Here's how the part is built. I have some questions about the finished solid (model axes, mm). A direction names the side the tool comes from. Round coordinates to 2 decimals unless told otherwise and drop trailing zeros. Loops run counter-clockwise (first coordinate to the right, second up) from the corner with the lowest first, then second, coordinate; pieces in that order, holes last. Notation, with made-up numbers: (54, 9.25) -> (69, 9.25) arc R17 cw to (69, 33.25) -> close; hole circle Ø6 at (28.5, 6). An arc over 180 degrees is marked (long way). Use one line per item in the form item = value. Start each with the question number.
Item 1: I'm going to push flat-ended pins straight in: pin 1 Ø2 at (x, z) = (22, 165) entering from -Y; pin 2 Ø14 at (x, z) = (119, 127.5) entering from -Y; pin 3 Ø3 at (x, z) = (64.5, 83.5) entering from -Y. Where does each tip first touch, or does it pass through?
Item 2: If we section it at B-B (z = 110.5): Write out the boundary of the cut face in (x, y).
Item 3: For faces 1 (the face through (-119, -32.5, 135)), 2 (the face through (-119, 32.5, 135)), 3 (the face through (118, -32.5, 135)), 4 (the face through (118, 32.5, 135)), which set-ups out of +Z, -Z, +X, -X, +Y, -Y let a thin tool reach every point of the face, with its end or its side?
Item 4: If I drill on L1, parallel to X at y = 0, z = 72.5; L2, parallel to Y at x = 1, z = 78 (3 decimals); L3, parallel to Y at x = 5, z = 12, over which ranges is the centre line in solid material (lowest first)? Write a range as [from, to].
Item 5: If we section it at C-C (z = 83): Write out the boundary of the cut face in (x, y), then the cut area to 3 significant figures.
Item 6: Thinking about a two-plate mould opening in X: for faces 5 (the face through (126, 0, 155)), 6 (the face through (-142.5, 0, 135)), 7 (the face through (96.5, 34.96, 134.51)), which applies, released by +X, released by -X, zero draft, split by the parting line, or undercut?
Item 7: If we section it at A-A (y = 0): Write out the boundary of the cut face in (x, z), then the cut area to 3 significant figures.
```python
from build123d import *

# Parameters (mm, degrees)
F0_R          = 100
F1_DEPTH      = 185
F2_W          = 62.5
F2_H          = 40
F3_DEPTH      = 32.5
F3_DEPTH_BACK = 32.5
F4_R          = 10
F5_R          = 5
F6_R          = 15


with BuildPart() as f1:
    # F0 (on Top) → F1 (new body)
    with BuildSketch(Plane.XY):
        Circle(F0_R)
    extrude(amount=F1_DEPTH)

    # F2 (on Front) → F3 (join, two sides)
    with BuildSketch(Plane.XZ) as f3_sk:
        with Locations((-111.25, 135)):
            Rectangle(F2_W, F2_H)
        with Locations((111.25, 135)):
            Rectangle(F2_W, F2_H)
    extrude(amount=F3_DEPTH)
    extrude(f3_sk.sketch, amount=-F3_DEPTH_BACK)

    # F4
    f4_edges = [f1.edges().sort_by_distance(p)[0] for p in [
        (-142.5, -32.5, 135),
        (-142.5, 32.5, 135),
        (142.5, -32.5, 135),
        (142.5, 32.5, 135),
    ]]
    fillet(f4_edges, radius=F4_R)

    # F5
    f5_edges = [f1.edges().sort_by_distance(p)[0] for p in [
        (-100, 0, 185),
    ]]
    fillet(f5_edges, radius=F5_R)

    # F6
    f6_edges = [f1.edges().sort_by_distance(p)[0] for p in [
        (100, 0, 167.5),
        (-100, 0, 180),
        (98.633514, -16.47513, 155),
        (94.571402, -32.5, 135),
        (98.633514, 16.47513, 155),
        (98.633514, -16.47513, 115),
        (94.571402, 32.5, 135),
        (100, 0, 57.5),
        (98.633514, 16.47513, 115),
        (-100, 0, 0),
        (-94.571402, -32.5, 135),
        (-100, 0, 115),
        (-94.571402, 32.5, 135),
        (-100, 0, 155),
    ]]
    fillet(f6_edges, radius=F6_R)


solid = f1.part
```
Values found:
q1.pin_1 = -97.77
q1.pin_2 = -32.5
q1.pin_3 = -77.66
q2.outline = (-98.66, -33.78) arc R15 cw to (-91.07, -41.3) arc R100 ccw to (91.07, -41.3) arc R15 cw to (98.66, -33.78) arc R104.29 ccw to (98.66, 33.78) arc R15 cw to (91.07, 41.3) arc R100 ccw to (-91.07, 41.3) arc R15 cw to (-98.66, 33.78) arc R104.29 ccw to start
q3.face_1 = +Z, -Z, -X, -Y
q3.face_2 = +Z, -Z, -X, +Y
q3.face_3 = +Z, -Z, +X, -Y
q3.face_4 = +Z, -Z, +X, +Y
q4.L1 = [-100, 100]
q4.L2 = [-99.995, 99.995]
q4.L3 = [-99.57, 99.57]
q5.outline = circle Ø200 at (0, 0)
q5.area = 31,400 mm2
q6.face_5 = zero draft
q6.face_6 = released by -X
q6.face_7 = released by +X
q7.outline = (-142.5, 115) -> (-115, 115) arc R15 cw to (-100, 100) -> (-100, 15) arc R15 ccw to (-85, 0) -> (85, 0) arc R15 ccw to (100, 15) -> (100, 100) arc R15 cw to (115, 115) -> (142.5, 115) -> (142.5, 155) -> (115, 155) arc R15 cw to (100, 170) -> (100, 180) arc R5 ccw to (95, 185) -> (-95, 185) arc R5 ccw to (-100, 180) -> (-100, 170) arc R15 cw to (-115, 155) -> (-142.5, 155) -> close
q7.area = 40,500 mm2
